Input: dimensioned drawing with shaded views. Units: mm. Origin: part minimum x, y, z. Give positions to 0.01 mm unless a question says otherwise; leave off trailing zeros. Write each loop counter-clockwise with the first axis right and the second up, starting at its lowest first coordinate (ties: lowest second). Pieces come first, ordered by that corner, then holes.
Q1. Section C-C (z = 1.2). Return the cut outline in (x, y), plus the area to 3 significant figures.
Q2. Pin query (flat end, axial travel): pin 1 Ø3.5 at (x, y) = (2.75, 5.25) entering from -Z; pin 2 Ø11 at (x, y) = (15.5, 17) entering from +Z; pin 3 Ø0.8 at (x, z) = (26, 1.5) entering from -Y; pin 4 Ø1.1 at (y, z) = (2.5, 2.5) entering from +X. Return the tip coordinate at first contact, or that it passes through.
Q3. Line query: line 1 (Y direction, x = 2.75, z = 1.35); line 2 (X direction, y = 36, z = 0.9); line 3 (Z direction, x = 17.5, y = 22.5). Output: solid intervals per line, ascending.
Q4. Section A-A (x = 2.75). Return the cut outline in (y, z).
Q5. Section B-B (y = 35.75). Return the cut outline in (x, z).
Q6. Section D-D (x = 18). Return the cut outline in (y, z), plus the area to 3 significant figures.
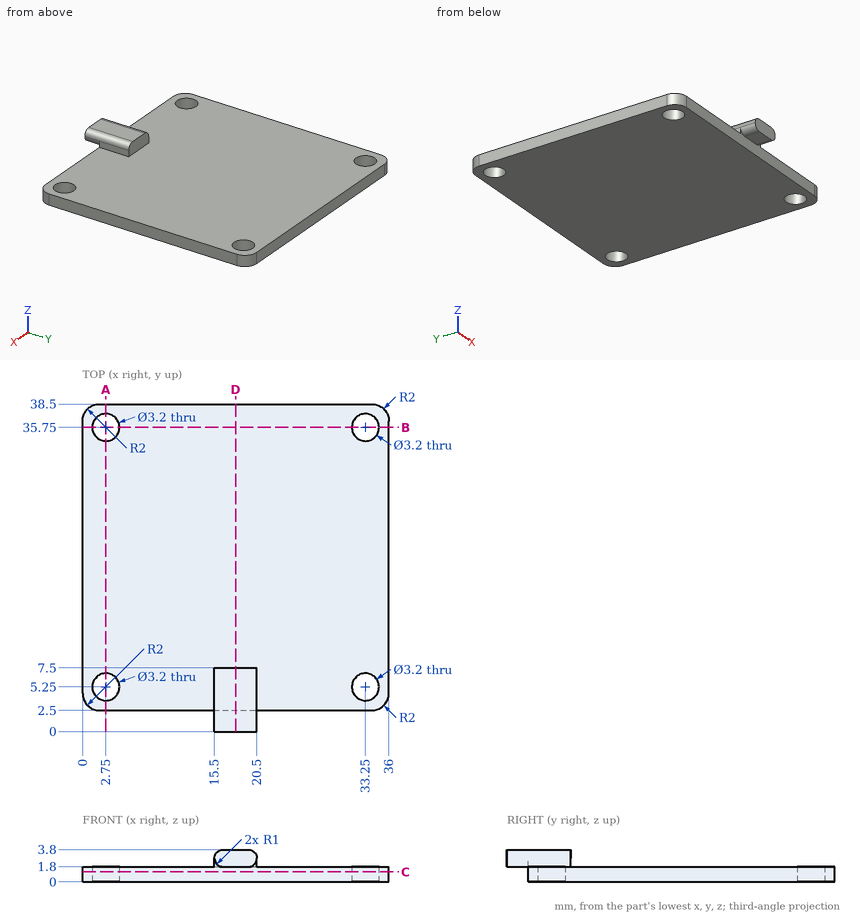
Computed:
1. outline: (0, 4.5) arc R2 ccw to (2, 2.5) - (34, 2.5) arc R2 ccw to (36, 4.5) - (36, 36.5) arc R2 ccw to (34, 38.5) - (2, 38.5) arc R2 ccw to (0, 36.5) - close; hole circle Ø3.2 at (2.75, 5.25); hole circle Ø3.2 at (2.75, 35.75); hole circle Ø3.2 at (33.25, 5.25); hole circle Ø3.2 at (33.25, 35.75)
1. area: 1,260 mm2
2. pin 1: stops at z = 0
2. pin 2: stops at z = 1.8
2. pin 3: stops at y = 2.5
2. pin 4: stops at x = 20.5
3. line 1: y = 2.5 to 3.65, 6.85 to 34.15, 37.35 to 38.5
3. line 2: x = 0 to 1.17, 4.33 to 31.67, 34.83 to 36
3. line 3: z = 0 to 1.8
4. outline: (2.5, 0) - (3.65, 0) - (3.65, 1.8) - (2.5, 1.8) - close; (6.85, 0) - (34.15, 0) - (34.15, 1.8) - (6.85, 1.8) - close; (37.35, 0) - (38.5, 0) - (38.5, 1.8) - (37.35, 1.8) - close
5. outline: (0, 0) - (1.15, 0) - (1.15, 1.8) - (0, 1.8) - close; (4.35, 0) - (31.65, 0) - (31.65, 1.8) - (4.35, 1.8) - close; (34.85, 0) - (36, 0) - (36, 1.8) - (34.85, 1.8) - close
6. outline: (0, 1.8) - (2.5, 1.8) - (2.5, 0) - (38.5, 0) - (38.5, 1.8) - (7.5, 1.8) - (7.5, 3.8) - (0, 3.8) - close
6. area: 79.8 mm2
